The model under review builds one solid part; all positions refer to its coordinate system, in mm. A direction names the side the tool comes from. Round coordinates to 2 decimals unless told otherwise and drop trailing zeros. Order: outer loops, then holes, each group sorted by start corner. A loop starts at its lowest first (then second) coordinate and runs counter-clockwise, first axis right, second up. Notation, with made-up numbers: (10, -35.75) - (40, -35.75) arc R34 cw to (40, -5.75) - close; hole circle Ø6 at (-19, 21). An arc over 180 degrees is marked (long way). One line per question, with ' | ' between items. Start each with the question number.
Item 1: Insertion check: pin 1 Ø22.5 at (x, y) = (33.5, 46) entering from -Z; pin 2 Ø5 at (x, z) = (34, -9) entering from +Y; pin 3 Ø1 at (x, z) = (17.5, -13) entering from +Y. Each pin has a flat end and moves straight along its axis. Give the tip position at first contact, or say it passes through.
Item 2: Add section B-B on x = 38.5. State the section outline as (y, z) points, and give its area (3 significant figures).
Item 3: For L1, parallel to X at y = 61, z = -4.75 (3 decimals); L2, parallel to Z at x = 8.5, y = 44; L3, parallel to Y at x = 25.5, z = -8.5, list the stretches that pass through material, from the lowest coordinate up. Write a range as [from, to].
Item 4: Draft analysis for pull direction X (two halves, no side actions). For faces 4 (the face through (30.226, 41.467, -2.576)), 5 (the face through (44.958, 41, -4)), 6 (the face through (22.16, 5.69, -5.66)), state which applies: +X half, -X half, draft (parallel to the pull), parting line (faces both ways), or undercut.
Item 5: Add section A-A on y = 74. State the section outline as (x, z) points, and give its area (3 significant figures).
Item 6: Add section D-D on z = -3.5. State how many separate pieces and enclosed holes the cut face has, and give its area (3 significant figures).
Item 7: Add section C-C on y = 36.5. State the section outline as (x, z) points, and give its area (3 significant figures).
Item 8: Tool access review of faces 1 (the face through (22, 48, 0)), 2 (the face through (2.489, 71, -3)), 3 (the face through (27, 49, -5.08)): name each direction out of +Z, -Z, +X, -X, +Y, -Y from which nothing blocks a thin tool from reaching the whole face with its end or side.
from build123d import *

# Parameters (mm, degrees)
BOSS_EXTRUDE6_DEPTH = 44.958
SKETCH12_R          = 4.953
SKETCH12_R_2        = 2.54
CUT_EXTRUDE1_DEPTH  = 102.639997127
FILLET4_R           = 2.032
FILLET5_R           = 2.032
FILLET6_R           = 2.032
FILLET7_R           = 2.032
SKETCH15_R          = 2.54
CUT_EXTRUDE2_DEPTH  = 99.086762695


with BuildPart() as part:
    # Sketch6 → Boss-Extrude6 (new body)
    with BuildSketch(Plane(origin=(0, 0, 0), x_dir=(0, 0, -1), z_dir=(1, 0, 0))):
        with BuildLine():
            Line((0, 7.112), (0, 89.916))
            Line((0, 89.916), (5.08, 89.916))
            Line((5.08, 89.916), (5.08, 7.112))
            ThreePointArc((5.08, 7.112), (5.675159021, 5.675159021), (7.112, 5.08))
            Line((7.112, 5.08), (20.066, 5.08))
            Line((20.066, 5.08), (20.066, 0))
            Line((20.066, 0), (7.112, 0))
            ThreePointArc((7.112, 0), (2.083056572, 2.083056572), (0, 7.112))
        make_face()
    extrude(amount=BOSS_EXTRUDE6_DEPTH)

    # Sketch12 → Cut-Extrude1 (cut, through all)
    with BuildSketch(Plane(origin=(0, 0, -5.08), x_dir=(-1, 0, 0), z_dir=(0, 0, -1))):
        with Locations((-34.9504, 79.9592)):
            Circle(SKETCH12_R)
        with Locations((-14.9606, 79.9592)):
            Circle(SKETCH12_R)
        with Locations((-14.9606, 59.9694)):
            Circle(SKETCH12_R)
        with Locations((-14.9606, 39.9796)):
            Circle(SKETCH12_R)
        with Locations((-14.9606, 19.9898)):
            Circle(SKETCH12_R)
        with Locations((-34.9504, 59.9694)):
            Circle(SKETCH12_R)
        with Locations((-34.9504, 39.9796)):
            Circle(SKETCH12_R)
        with Locations((-34.9504, 19.9898)):
            Circle(SKETCH12_R)
        with Locations((-19.9136, 49.9745)):
            Circle(SKETCH12_R_2)
        with Locations((-19.9136, 69.9643)):
            Circle(SKETCH12_R_2)
        with Locations((-19.9136, 29.9847)):
            Circle(SKETCH12_R_2)
        with BuildLine():
            Line((-2.4892, 74.9046), (-2.4892, 67.0306))
            ThreePointArc((-2.4892, 67.0306), (-5.0292, 64.4906), (-7.5692, 67.0306))
            Line((-7.5692, 67.0306), (-7.5692, 74.9046))
            ThreePointArc((-7.5692, 74.9046), (-5.0292, 77.4446), (-2.4892, 74.9046))
        make_face()
        with BuildLine():
            Line((-2.4892, 55.0418), (-2.4892, 47.1678))
            ThreePointArc((-2.4892, 47.1678), (-5.0292, 44.6278), (-7.5692, 47.1678))
            Line((-7.5692, 47.1678), (-7.5692, 55.0418))
            ThreePointArc((-7.5692, 55.0418), (-5.0292, 57.5818), (-2.4892, 55.0418))
        make_face()
        with BuildLine():
            Line((-2.4892, 35.179), (-2.4892, 27.305))
            ThreePointArc((-2.4892, 27.305), (-5.0292, 24.765), (-7.5692, 27.305))
            Line((-7.5692, 27.305), (-7.5692, 35.179))
            ThreePointArc((-7.5692, 35.179), (-5.0292, 37.719), (-2.4892, 35.179))
        make_face()
    extrude(amount=-CUT_EXTRUDE1_DEPTH, mode=Mode.SUBTRACT)

    # Fillet4
    fillet4_edges = [part.edges().sort_by_distance(p)[0] for p in [
        (44.958, 89.916, -2.54),
    ]]
    fillet(fillet4_edges, radius=FILLET4_R)

    # Fillet5
    fillet5_edges = [part.edges().sort_by_distance(p)[0] for p in [
        (44.958, 2.54, -20.066),
    ]]
    fillet(fillet5_edges, radius=FILLET5_R)

    # Fillet6
    fillet6_edges = [part.edges().sort_by_distance(p)[0] for p in [
        (0, 2.54, -20.066),
    ]]
    fillet(fillet6_edges, radius=FILLET6_R)

    # Fillet7
    fillet7_edges = [part.edges().sort_by_distance(p)[0] for p in [
        (0, 89.916, -2.54),
    ]]
    fillet(fillet7_edges, radius=FILLET7_R)

    # Sketch15 → Cut-Extrude2 (cut, through all)
    with BuildSketch(Plane(origin=(0, 5.08, 0), x_dir=(1, 0, 0), z_dir=(0, 1, 0))):
        with Locations(Location((15.0114, 14.986, 0), (0, 0, 270))):
            Circle(SKETCH15_R)
        with Locations(Location((35.0012, 14.986, 0), (0, 0, 270))):
            Circle(SKETCH15_R)
    extrude(amount=-CUT_EXTRUDE2_DEPTH, mode=Mode.SUBTRACT)


solid = part.part
Determined:
1) pin 1: z = -5.08 | pin 2: y = 5.17 | pin 3: y = 5.08
2) outline: (0, -20.07) - (5.08, -20.07) - (5.08, -7.11) arc R2.03 cw to (7.11, -5.08) - (16.54, -5.08) - (16.54, 0) - (7.11, 0) arc R7.11 ccw to (0, -7.11) - close; (23.44, -5.08) - (36.53, -5.08) - (36.53, 0) - (23.44, 0) - close; (43.43, -5.08) - (56.52, -5.08) - (56.52, 0) - (43.43, 0) - close; (63.42, -5.08) - (76.5, -5.08) - (76.5, 0) - (63.42, 0) - close; (83.41, -5.08) - (89.92, -5.08) - (89.92, 0) - (83.41, 0) - close | area: 383 mm2
3) L1: [0, 10.116], [19.805, 30.106], [39.795, 44.958] | L2: [-5.08, 0] | L3: [0, 5.08]
4) face 4: undercut | face 5: +X half | face 6: draft
5) outline: (0, -5.08) - (2.49, -5.08) - (2.49, 0) - (0, 0) - close; (7.57, -5.08) - (44.96, -5.08) - (44.96, 0) - (7.57, 0) - close | area: 203 mm2
6) separate pieces: 1 | enclosed holes: 14 | area: 3,140 mm2
7) outline: (0, -5.08) - (2.86, -5.08) - (2.86, 0) - (0, 0) - close; (7.2, -5.08) - (11.44, -5.08) - (11.44, 0) - (7.2, 0) - close; (18.49, -5.08) - (31.43, -5.08) - (31.43, 0) - (18.49, 0) - close; (38.48, -5.08) - (44.96, -5.08) - (44.96, 0) - (38.48, 0) - close | area: 135 mm2
8) face 1: +Z, +X, -X, +Y, -Y | face 2: +Z, -Z | face 3: -Z, +X, -X, +Y
